Autodesk Inventor part; units mm, degrees
ref_plane "YZ Plane" through (0, 0, 0) normal (1, 0, 0) x (0, 1, 0)
ref_plane "XZ Plane" through (0, 0, 0) normal (0, 1, 0) x (-1, 0, 0)
ref_plane "XY Plane" through (0, 0, 0) normal (0, 0, 1) x (1, 0, 0)
sketch "Sketch1" plane through (0, 0, 0) normal (0, 1, 0) x (-1, 0, 0)
  circle A0 centre (0, 0) radius 3.5 construction
  circle A1 centre (0, 0) radius 5
  line L0 (3.5, -2.0207) -> (0, -4.0415)
  line L1 (0, -4.0415) -> (-3.5, -2.0207)
  line L2 (-3.5, -2.0207) -> (-3.5, 2.0207)
  line L3 (-3.5, 2.0207) -> (0, 4.0415)
  line L4 (0, 4.0415) -> (3.5, 2.0207)
  line L5 (3.5, 2.0207) -> (3.5, -2.0207)
  point P0 (3.5, 0)
  dimension "d0" = 7
  dimension "d1" = 10
extrude "Extrusion1" add sketch "Sketch1" along normal blind 8
properties part number "8mm Rex Spacer"
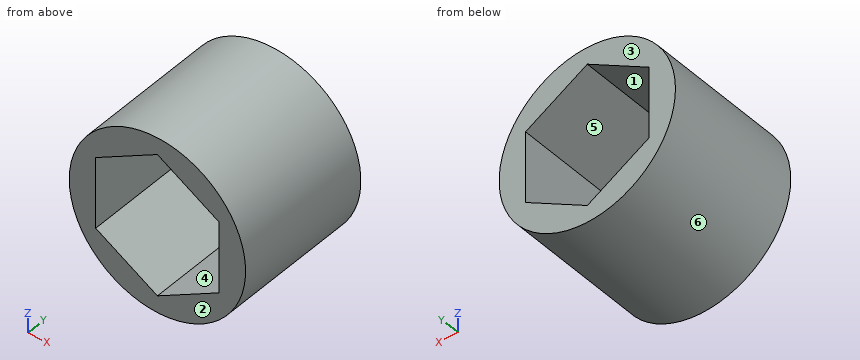
Verification items for the finished model (mm, model axes). Face numbers are marked on the shaded views. A direction names the side the tool comes from. Round coordinates to 2 decimals unless told otherwise and drop trailing zeros. Write each loop counter-clockwise with the first axis right and the second up, starting at its lowest first coordinate (ties: lowest second). Pieces come first, ordered by that corner, then holes.
(1) Material ranges on line 1 (X direction, y = 2, z = 3.5); line 2 (X direction, y = 1.5, z = -1.75); line 3 (Z direction, x = -3, y = 5), recorded low to high.
Returned:
line 1: x = -3.57 to -0.94, 0.94 to 3.57
line 2: x = -4.68 to -3.5, 3.5 to 4.68
line 3: z = -4 to -2.31, 2.31 to 4
(2) Depth check by flat-ended pin: pin 1 Ø3 at (x, y) = (3, 3) entering from +Z; pin 2 Ø3 at (x, y) = (-2.5, 5.5) entering from -Z; pin 3 Ø1 at (x, y) = (4, 5) entering from +Z. Enter the tip coordinate at first touch or a pass-through.
Returned:
pin 1: stops at z = 4.77
pin 2: stops at z = -4.9
pin 3: stops at z = 3.57
(3) Section check B-B (z = 0). Enter the section's corners in (x, y), plus the area to 3 significant figures.
Returned:
outline: (-5, 0) - (-3.5, 0) - (-3.5, 8) - (-5, 8) - close; (3.5, 0) - (5, 0) - (5, 8) - (3.5, 8) - close
area: 24.0 mm2
(4) Mould release check, pull along Z, two halves, no side actions. Record for the marked faces 3, 4, 5 and 6: pulls with the +Z half, pulls with the -Z half, needs draft (parallel to the pull), parting line crosses it, or undercut.
Returned:
face 3: needs draft
face 4: undercut
face 5: undercut
face 6: parting line crosses it
(5) Section check C-C (x = 2). Enter the section's corners in (y, z).
Returned:
outline: (0, -4.58) - (8, -4.58) - (8, -2.89) - (0, -2.89) - close; (0, 2.89) - (8, 2.89) - (8, 4.58) - (0, 4.58) - close
(6) Section check A-A (y = 7.25). Enter the section's corners in (x, z).
Returned:
outline: circle Ø10 at (0, 0); hole (-3.5, -2.02) - (0, -4.04) - (3.5, -2.02) - (3.5, 2.02) - (0, 4.04) - (-3.5, 2.02) - close
(7) Access from +Z, -Z, +X, -X, +Y, -Y to the whole of each face (thin tool, end or side, straight path). Record for the marked faces 1 and 2.
Returned:
face 1: +Y, -Y
face 2: +Z, -Z, +X, -X, -Y
